from build123d import *

# Parameters (mm, degrees)
SKETCH_1_R          = 1
EXTRUDE_1_DEPTH     = 4
SKETCH_2_W          = 34
SKETCH_2_H          = 2
EXTRUDE_2_DEPTH     = 36
SKETCH_3_R          = 0.95
SKETCH_3_W          = 12
SKETCH_3_H          = 14.169811535
CUT_EXTRUDE_1_DEPTH = 3
EXTRUDE_START       = 2
SKETCH_4_R          = 2.2
SKETCH_4_R_2        = 0.95
EXTRUDE_3_DEPTH     = 2
FILLET_1_R          = 5
EXTRUDE_5_DEPTH     = 6


with BuildPart() as part:
    # Эскиз1 → Бобышка-Вытянуть1 (new body)
    with BuildSketch(Plane.XY):
        with BuildLine():
            Line((-17, -11.5), (17, -11.5))
            Line((17, -11.5), (17, 11.5))
            Line((17, 11.5), (2, 11.5))
            Line((2, 11.5), (2, 8.031128874))
            ThreePointArc((2, 8.031128874), (0, -0.5), (-2, 8.031128874))
            Line((-2, 8.031128874), (-2, 11.5))
            Line((-2, 11.5), (-17, 11.5))
            Line((-17, 11.5), (-17, -11.5))
        make_face()
        with Locations((-13.5, 8.5)):
            Circle(SKETCH_1_R, mode=Mode.SUBTRACT)
        with Locations((13.5, 8.5)):
            Circle(SKETCH_1_R, mode=Mode.SUBTRACT)
        with Locations((-13.5, -2.5)):
            Circle(SKETCH_1_R, mode=Mode.SUBTRACT)
        with Locations((13.5, -2.5)):
            Circle(SKETCH_1_R, mode=Mode.SUBTRACT)
    extrude(amount=EXTRUDE_1_DEPTH)

    # Эскиз2 → Бобышка-Вытянуть2 (add)
    with BuildSketch(Plane(origin=(0, 0, 0), x_dir=(-1, 0, 0), z_dir=(0, 0, -1))):
        with Locations((0, -10.5)):
            Rectangle(SKETCH_2_W, SKETCH_2_H)
    extrude(amount=EXTRUDE_2_DEPTH)

    # Эскиз3 → Вырез-Вытянуть1 (cut)
    with BuildSketch(Plane.XZ.offset(11.5)):
        with Locations(Location((11.75, -7, 0), (0, 0, 270))):
            Circle(SKETCH_3_R)
        with Locations(Location((11.75, -30.5, 0), (0, 0, 270))):
            Circle(SKETCH_3_R)
        with Locations(Location((-11.75, -30.5, 0), (0, 0, 270))):
            Circle(SKETCH_3_R)
        with Locations(Location((-11.75, -7, 0), (0, 0, 270))):
            Circle(SKETCH_3_R)
        with Locations((0, -10.084905768)):
            Rectangle(SKETCH_3_W, SKETCH_3_H)
    extrude(amount=-CUT_EXTRUDE_1_DEPTH, mode=Mode.SUBTRACT)

    # Эскиз4 → Бобышка-Вытянуть3 (add)
    # profile 1 of 4: a face of its own
    with BuildSketch(Plane.XZ.offset(11.5).offset(EXTRUDE_START)):
        with Locations(Location((11.75, -7, 0), (0, 0, 90))):
            Circle(SKETCH_4_R)
        with Locations(Location((11.75, -7, 0), (0, 0, 270))):
            Circle(SKETCH_4_R_2, mode=Mode.SUBTRACT)
    # profile 2 of 4: a face of its own
    with BuildSketch(Plane.XZ.offset(11.5).offset(EXTRUDE_START)):
        with Locations(Location((11.75, -30.5, 0), (0, 0, 90))):
            Circle(SKETCH_4_R)
        with Locations(Location((11.75, -30.5, 0), (0, 0, 270))):
            Circle(SKETCH_4_R_2, mode=Mode.SUBTRACT)
    # profile 3 of 4: a face of its own
    with BuildSketch(Plane.XZ.offset(11.5).offset(EXTRUDE_START)):
        with Locations(Location((-11.75, -7, 0), (0, 0, 90))):
            Circle(SKETCH_4_R)
        with Locations(Location((-11.75, -7, 0), (0, 0, 270))):
            Circle(SKETCH_4_R_2, mode=Mode.SUBTRACT)
    # profile 4 of 4: a face of its own
    with BuildSketch(Plane.XZ.offset(11.5).offset(EXTRUDE_START)):
        with Locations(Location((-11.75, -30.5, 0), (0, 0, 90))):
            Circle(SKETCH_4_R)
        with Locations(Location((-11.75, -30.5, 0), (0, 0, 270))):
            Circle(SKETCH_4_R_2, mode=Mode.SUBTRACT)
    extrude(amount=-EXTRUDE_3_DEPTH)

    # Скругление1
    fillet_1_edges = [part.edges().sort_by_distance(p)[0] for p in [
        (17, -10.5, -36),
        (-17, -10.5, -36),
    ]]
    fillet(fillet_1_edges, radius=FILLET_1_R)

    # Эскиз5 → Бобышка-Вытянуть5 (add)
    with BuildSketch(Plane.XZ.offset(11.5)):
        Polygon((14, -32.75), (-14, -32.75), (-14, -4.75), (-6, -4.75), (-6, -3.25), (-15.5, -3.25), (-15.5, -34.25), (15.5, -34.25), (15.5, -3.25), (6, -3.25), (6, -4.75), (14, -4.75), align=None)
    extrude(amount=EXTRUDE_5_DEPTH)


solid = part.part
Design review of the part built by this model. Coordinates are the model's own, in mm. A direction names the side the tool comes from. Round coordinates to 2 decimals unless told otherwise and drop trailing zeros. Write each loop counter-clockwise with the first axis right and the second up, starting at its lowest first coordinate (ties: lowest second). Pieces come first, ordered by that corner, then holes. Notation, with made-up numbers: (26.5, -16.5) -> (37.5, -16.5) arc R7 cw to (37.5, -3.5) -> close; hole circle Ø9 at (12, -5). An arc over 180 degrees is marked (long way). One line per item, written item: value. Start each with the question number.
Q1. Add section C-C (x = 0). Give the boundary of the cut face in (y, z).
Q2. Insertion check: P1, Ø2, axis at x = 2, z = -3, coming from the -Y side; P2, Ø3, axis at x = -2, y = 1, coming from the +Z side; P3, Ø3, axis at y = -15, z = -21, coming from the +X side; P4, Ø1, axis at y = -8, z = -5.5, coming from the -X side. Each pin has a flat end and moves straight along its axis. Give the tip position at first contact, or say it passes through.
Q3. Tool access review of faces 1 (the face through (0, -11.5, -19)), 2 (the face through (-11, -14, -3.25)), 3 (the face through (-2, 10, 2)), 4 (the face through (0, -9.5, -18)): name each direction out of +Z, -Z, +X, -X, +Y, -Y from which nothing blocks a thin tool from reaching the whole face with its end or side.
Q4. To check wall thickness, follow probe 1 along Y at (x, z) = (-13.5, 1.9); probe 2 along X at (y, z) = (-10.6, -30.5); probe 3 along X at (y, z) = (4, 1.65). State the ranges of each line that lie inside material, in increasing order.
Q5. Add section A-A (z = -30.5). Give the boundary of the cut face in (x, y).
Q6. The part is to be moulded in two halves that separate along X. For faces 5 (the face through (14.454, -2.2, 1.972)), 6 (the face through (0, -14, -34.25)), 7 (the face through (-17, -5, 1)), say which applies: pulls with the +X half, pulls with the -X half, needs draft (parallel to the pull), parting line crosses it, or undercut.
Q7. Add section B-B (y = -12). State how many separate pieces and enclosed holes the cut face has, then the cut area to 3 significant figures.
Response:
1. outline: (-17.5, -34.25) -> (-11.5, -34.25) -> (-11.5, -36) -> (-9.5, -36) -> (-9.5, -17.17) -> (-11.5, -17.17) -> (-11.5, -32.75) -> (-17.5, -32.75) -> close; (-11.5, -3) -> (-9.5, -3) -> (-9.5, 0) -> (-0.5, 0) -> (-0.5, 4) -> (-11.5, 4) -> close
2. P1: stops at y = -11.5
2. P2: stops at z = 4
2. P3: stops at x = 15.5
2. P4: passes through
3. face 1: -Y
3. face 2: +Z, +X, -X, -Y
3. face 3: +Z, -Z, +Y
3. face 4: -Z, +X, -X, +Y
4. probe 1: y = -11.5 to -3.5, -1.5 to 7.5, 9.5 to 11.5
4. probe 2: x = -17 to -12.7, -10.8 to 10.8, 12.7 to 17
4. probe 3: x = -17 to -4.5, 4.5 to 17
5. outline: (-17, -11.5) -> (-15.5, -11.5) -> (-15.5, -17.5) -> (-14, -17.5) -> (-14, -11.5) -> (-13.95, -11.5) -> (-13.95, -13.5) -> (-12.7, -13.5) -> (-12.7, -9.5) -> (-17, -9.5) -> close; (-10.8, -13.5) -> (-9.55, -13.5) -> (-9.55, -11.5) -> (9.55, -11.5) -> (9.55, -13.5) -> (10.8, -13.5) -> (10.8, -9.5) -> (-10.8, -9.5) -> close; (12.7, -13.5) -> (13.95, -13.5) -> (13.95, -11.5) -> (14, -11.5) -> (14, -17.5) -> (15.5, -17.5) -> (15.5, -11.5) -> (17, -11.5) -> (17, -9.5) -> (12.7, -9.5) -> close
6. face 5: undercut
6. face 6: needs draft
6. face 7: pulls with the -X half
7. separate pieces: 5
7. enclosed holes: 4
7. area: 208 mm^2
